Here's how the part is built. I have some questions about the finished solid (model axes, mm). A direction names the side the tool comes from. Give positions to 0.01 mm unless a question says otherwise; leave off trailing zeros. Order: outer loops, then holes, each group sorted by start corner. A loop starts at its lowest first (then second) coordinate and runs counter-clockwise, first axis right, second up. Notation, with made-up numbers: M 0,81.25 L 11,81.25 A21 cw 11,111.25 Z; hole C 76,-31 d6. An arc over 180 degrees is marked long. Use CSV: the item, a comma, the result in double quotes. Start each with the question number.
```python
from build123d import *

# Parameters (mm, degrees)
SKETCH1_W             = 40.386
SKETCH1_H             = 20.447
BOSS_EXTRUDE1_DEPTH   = 15.4178
FILLET1_R             = 0.508
F_2_CLEARANCE_HOLE1_D = 2.2606
SKETCH8_R             = 1.524
CUT_EXTRUDE2_DEPTH    = 1.905
SKETCH6_R             = 8.5725
CUT_EXTRUDE5_DEPTH    = 28.385867854
CUT_EXTRUDE6_DEPTH    = 28.385867854
SKETCH11_W            = 37.9222
SKETCH11_H            = 17.9832
SKETCH11_R            = 1.1303
CUT_EXTRUDE7_DEPTH    = 1.5621


with BuildPart() as part:
    # Sketch1 → Boss-Extrude1 (new body)
    with BuildSketch(Plane(origin=(0, 0, 0), x_dir=(1, 0, 0), z_dir=(0, 1, 0))):
        Rectangle(SKETCH1_W, SKETCH1_H)
    extrude(amount=BOSS_EXTRUDE1_DEPTH)

    # Fillet1
    fillet1_edges = [part.edges().sort_by_distance(p)[0] for p in [
        (20.193, 7.7089, 10.2235),
        (-20.193, 7.7089, 10.2235),
        (-20.193, 7.7089, -10.2235),
        (20.193, 7.7089, -10.2235),
    ]]
    fillet(fillet1_edges, radius=FILLET1_R)

    # #2 Clearance Hole1 (through all)
    with Locations(Plane(origin=(0, 15.4178, 0), x_dir=(1, 0, 0), z_dir=(0, 1, 0))):
        with Locations((17.57045, -7.5311), (-17.57045, 7.5311), (-17.57045, -7.5311), (17.57045, 7.5311)):
            Hole(F_2_CLEARANCE_HOLE1_D / 2)

    # Sketch8 → Cut-Extrude2 (cut)
    with BuildSketch(Plane(origin=(0, 15.4178, 0), x_dir=(1, 0, 0), z_dir=(0, 1, 0))):
        with Locations(Location((-17.57045, -7.5311, 0), (0, 0, 270))):
            Circle(SKETCH8_R)
        with Locations(Location((-17.57045, 7.5311, 0), (0, 0, 270))):
            Circle(SKETCH8_R)
        with Locations(Location((17.57045, 7.5311, 0), (0, 0, 270))):
            Circle(SKETCH8_R)
        with Locations(Location((17.57045, -7.5311, 0), (0, 0, 270))):
            Circle(SKETCH8_R)
    extrude(amount=-CUT_EXTRUDE2_DEPTH, mode=Mode.SUBTRACT)

    # Sketch6 → Cut-Extrude5 (cut, through all)
    with BuildSketch(Plane(origin=(0, 15.4178, 0), x_dir=(1, 0, 0), z_dir=(0, 1, 0))):
        with Locations(Location((-10.014739789, 0, 0), (0, 0, 270))):
            Circle(SKETCH6_R)
    extrude(amount=-CUT_EXTRUDE5_DEPTH, mode=Mode.SUBTRACT)

    # Sketch10 → Cut-Extrude6 (cut, through all)
    with BuildSketch(Plane(origin=(0, 15.4178, 0), x_dir=(1, 0, 0), z_dir=(0, 1, 0))):
        with BuildLine():
            Line((-4.548942478, 6.604), (-4.548942478, -6.604))
            Line((-4.548942478, -6.604), (-3.278942478, -6.604))
            Line((-3.278942478, -6.604), (-3.278942478, -8.0137))
            Line((-3.278942478, -8.0137), (14.99268629, -8.0137))
            ThreePointArc((14.99268629, -8.0137), (15.691232741, -5.701807515), (17.983482839, -4.941279084))
            Line((17.983482839, -4.941279084), (17.983482839, 4.870569671))
            ThreePointArc((17.983482839, 4.870569671), (15.641855904, 5.652392313), (14.921654991, 8.0137))
            Line((14.921654991, 8.0137), (-3.278942478, 8.0137))
            Line((-3.278942478, 8.0137), (-3.278942478, 6.604))
            Line((-3.278942478, 6.604), (-4.548942478, 6.604))
        make_face()
    extrude(amount=-CUT_EXTRUDE6_DEPTH, mode=Mode.SUBTRACT)

    # Sketch11 → Cut-Extrude7 (cut)
    with BuildSketch(Plane.XZ):
        Rectangle(SKETCH11_W, SKETCH11_H)
        with Locations(Location((17.57045, 7.5311, 0), (0, 0, 90))):
            Circle(SKETCH11_R, mode=Mode.SUBTRACT)
        with Locations(Location((-17.57045, 7.5311, 0), (0, 0, 90))):
            Circle(SKETCH11_R, mode=Mode.SUBTRACT)
        with Locations(Location((17.57045, -7.5311, 0), (0, 0, 90))):
            Circle(SKETCH11_R, mode=Mode.SUBTRACT)
        with Locations(Location((-17.57045, -7.5311, 0), (0, 0, 90))):
            Circle(SKETCH11_R, mode=Mode.SUBTRACT)
        with BuildLine():
            Line((14.921654991, -8.0137), (-3.278942478, -8.0137))
            Line((-3.278942478, -8.0137), (-3.278942478, -6.604))
            Line((-3.278942478, -6.604), (-4.548942478, -6.604))
            ThreePointArc((-4.548942478, -6.604), (-18.587239789, 0), (-4.548942478, 6.604))
            Line((-4.548942478, 6.604), (-3.278942478, 6.604))
            Line((-3.278942478, 6.604), (-3.278942478, 8.0137))
            Line((-3.278942478, 8.0137), (14.99268629, 8.0137))
            ThreePointArc((14.99268629, 8.0137), (15.691232741, 5.701807515), (17.983482839, 4.941279084))
            Line((17.983482839, 4.941279084), (17.983482839, -4.870569671))
            ThreePointArc((17.983482839, -4.870569671), (15.641855904, -5.652392313), (14.921654991, -8.0137))
        make_face(mode=Mode.SUBTRACT)
    extrude(amount=-CUT_EXTRUDE7_DEPTH, mode=Mode.SUBTRACT)


solid = part.part
```
Q1. Imagine slicing it at C-C, the plane y = 5.5. Please give me the cut outline in (x, z) (1 decimal), then the cut area to 3 significant figures.
Q2. Imagine slicing it at B-B, the plane x = 6. Please give me the cut outline in (y, z), then the cut area to 3 significant figures.
Q3. We'd pull the mould along Z, two halves only. Please class faces 6 (the face through (-4, 9, -6.604)), 7 (the face through (0, 8, 10.224)), 8 (the face through (0, 0, 10)): pulls with the +Z half, pulls with the -Z half, needs draft (parallel to the pull), parting line crosses it, or undercut.
Q4. For faces 1 (the face through (18.961, 1, 0)), 2 (the face through (0, 8, -10.224)), 3 (the face through (-3.279, 9, 7)), 4 (the face through (20.193, 8, 0)), 5 (the face through (16.64, 14.48, -8.74)), which set-ups out of +Z, -Z, +X, -X, +Y, -Y let a thin tool reach every point of the face, with its end or its side?
Q5. Imagine slicing it at A-A, the plane z = 0. Please give me the cut outline in (x, y), then the cut area to 3 significant figures.
Q6. For P1, Ø2.5, axis at x = -17.57, z = 7.53, coming from the +Y side; P2, Ø3.5, axis at x = -17.57, z = -7.53, coming from the -Y side; P3, Ø10, axis at x = -11.5, z = 0.5, coming from the -Y side, each with a flat end and sliding along its axis, tell me the tip position at first contact or that it passes through.
Q7. I need wall thicknesses on line 1 (X direction, y = 1.5, z = -4.5); line 2 (Z direction, x = -1.5, y = 2.5); line 3 (X direction, y = 8.5, z = -6.5). Which ranges of each line are inside material? Lowest first, please. Write a range as [from, to].
Reply:
1,outline,"M -20.2,-9.7 A0.5 ccw -19.7,-10.2 L 19.7,-10.2 A0.5 ccw 20.2,-9.7 L 20.2,9.7 A0.5 ccw 19.7,10.2 L -19.7,10.2 A0.5 ccw -20.2,9.7 Z; hole C -17.6,-7.5 d2.3; hole C -17.6,7.5 d2.3; hole M -4.5,-6.6 L -3.3,-6.6 L -3.3,-8 L 14.9,-8 A2.7 cw 18,-4.9 L 18,4.9 A2.6 cw 15,8 L -3.3,8 L -3.3,6.6 L -4.5,6.6 A8.6 ccw long Z; hole C 17.6,-7.5 d2.3; hole C 17.6,7.5 d2.3"
1,area,"266 mm^2"
2,outline,"M 0,-10.22 L 15.42,-10.22 L 15.42,-8.01 L 1.56,-8.01 L 1.56,-8.99 L 0,-8.99 Z; M 0,8.99 L 1.56,8.99 L 1.56,8.01 L 15.42,8.01 L 15.42,10.22 L 0,10.22 Z"
2,area,"65.1 mm^2"
3,face 6,"undercut"
3,face 7,"pulls with the +Z half"
3,face 8,"needs draft"
4,face 1,"-Y"
4,face 2,"-Z, +X, -X, +Y, -Y"
4,face 3,"+Y, -Y"
4,face 4,"+Z, -Z, +X, +Y, -Y"
4,face 5,"+Y"
5,outline,"M -20.19,0 L -18.96,0 L -18.96,1.56 L -18.59,1.56 L -18.59,15.42 L -20.19,15.42 Z; M 17.98,1.56 L 18.96,1.56 L 18.96,0 L 20.19,0 L 20.19,15.42 L 17.98,15.42 Z"
5,area,"56.7 mm^2"
6,P1,"stops at y = 13.51"
6,P2,"stops at y = 0"
6,P3,"passes through"
7,line 1,"x = [-20.19, -18.96], [18.96, 20.19]"
7,line 2,"z = [-10.22, -8.01], [8.01, 10.22]"
7,line 3,"x = [-20.19, -18.03], [-17.11, -15.6], [15.08, 17.11], [18.03, 20.19]"
